from build123d import *

# Parameters (mm, degrees)
F0_W      = 6.5
F0_H      = 6.5
F1_DEPTH  = 34
F2_R      = 1
F4_DEPTH  = 8
F5_W      = 15
F5_H      = 15
F5_R      = 4
F6_DEPTH  = 10
F8_DEPTH  = 4
F10_D     = 4
F10_DEPTH = 25
F10_TIP   = 1.2017212381
F11_R     = 2


with BuildPart() as f1:
    # F0 (on Top) → F1 (new body)
    with BuildSketch(Plane.XY):
        Rectangle(F0_W, F0_H)
    extrude(amount=F1_DEPTH)

    # F2
    f2_edges = [f1.edges().sort_by_distance(p)[0] for p in [
        (-3.25, 3.25, 17),
        (3.25, 3.25, 17),
        (3.25, -3.25, 17),
        (-3.25, -3.25, 17),
    ]]
    fillet(f2_edges, radius=F2_R)

    # F3 (on face) → F4 (join)
    with BuildSketch(Plane.XY.offset(34)):
        with BuildLine():
            ThreePointArc((3.25, 2.25), (3.249048632, 2.2936099868), (3.2461963381, 2.3371369952))
            ThreePointArc((3.2461963381, 2.3371369952), (2.8284271247, 2.8284271247), (2.3371369952, 3.2461963381))
            ThreePointArc((2.3371369952, 3.2461963381), (2.2936099868, 3.249048632), (2.25, 3.25))
            Line((2.25, 3.25), (-2.25, 3.25))
            ThreePointArc((-2.25, 3.25), (-2.2936099868, 3.249048632), (-2.3371369952, 3.2461963381))
            ThreePointArc((-2.3371369952, 3.2461963381), (-2.8284271247, 2.8284271247), (-3.2461963381, 2.3371369952))
            ThreePointArc((-3.2461963381, 2.3371369952), (-3.249048632, 2.2936099868), (-3.25, 2.25))
            Line((-3.25, 2.25), (-3.25, -2.25))
            ThreePointArc((-3.25, -2.25), (-3.249048632, -2.2936099868), (-3.2461963381, -2.3371369952))
            ThreePointArc((-3.2461963381, -2.3371369952), (-2.8284271247, -2.8284271247), (-2.3371369952, -3.2461963381))
            ThreePointArc((-2.3371369952, -3.2461963381), (-2.2936099868, -3.249048632), (-2.25, -3.25))
            Line((-2.25, -3.25), (2.25, -3.25))
            ThreePointArc((2.25, -3.25), (2.2936099868, -3.249048632), (2.3371369952, -3.2461963381))
            ThreePointArc((2.3371369952, -3.2461963381), (2.8284271247, -2.8284271247), (3.2461963381, -2.3371369952))
            ThreePointArc((3.2461963381, -2.3371369952), (3.249048632, -2.2936099868), (3.25, -2.25))
            Line((3.25, -2.25), (3.25, 2.25))
        make_face()
        with BuildLine():
            ThreePointArc((3.2461963381, -2.3371369952), (3.8068875313, -1.2278466206), (4, 0))
            ThreePointArc((4, 0), (3.8068875313, 1.2278466206), (3.2461963381, 2.3371369952))
            ThreePointArc((3.2461963381, 2.3371369952), (3.249048632, 2.2936099868), (3.25, 2.25))
            Line((3.25, 2.25), (3.25, -2.25))
            ThreePointArc((3.25, -2.25), (3.249048632, -2.2936099868), (3.2461963381, -2.3371369952))
        make_face()
        with BuildLine():
            ThreePointArc((2.25, 3.25), (2.2936099868, 3.249048632), (2.3371369952, 3.2461963381))
            ThreePointArc((2.3371369952, 3.2461963381), (0, 4), (-2.3371369952, 3.2461963381))
            ThreePointArc((-2.3371369952, 3.2461963381), (-2.2936099868, 3.249048632), (-2.25, 3.25))
            Line((-2.25, 3.25), (2.25, 3.25))
        make_face()
        with BuildLine():
            ThreePointArc((-2.3371369952, -3.2461963381), (0, -4), (2.3371369952, -3.2461963381))
            ThreePointArc((2.3371369952, -3.2461963381), (2.2936099868, -3.249048632), (2.25, -3.25))
            Line((2.25, -3.25), (-2.25, -3.25))
            ThreePointArc((-2.25, -3.25), (-2.2936099868, -3.249048632), (-2.3371369952, -3.2461963381))
        make_face()
        with BuildLine():
            ThreePointArc((-3.25, 2.25), (-3.249048632, 2.2936099868), (-3.2461963381, 2.3371369952))
            ThreePointArc((-3.2461963381, 2.3371369952), (-4, 0), (-3.2461963381, -2.3371369952))
            ThreePointArc((-3.2461963381, -2.3371369952), (-3.249048632, -2.2936099868), (-3.25, -2.25))
            Line((-3.25, -2.25), (-3.25, 2.25))
        make_face()
    extrude(amount=F4_DEPTH)

    # F5 (on face) → F6 (join)
    with BuildSketch(Plane.XY.offset(42)):
        Rectangle(F5_W, F5_H)
        Circle(F5_R, mode=Mode.SUBTRACT)
        Circle(F5_R)
    extrude(amount=F6_DEPTH)

    # F7 (on face) → F8 (cut)
    with BuildSketch(Plane.XY.offset(52)):
        Polygon((-3, 1.7320508076), (-3, -1.7320508076), (0, -3.4641016151), (3, -1.7320508076), (3, 1.7320508076), (0, 3.4641016151), align=None)
    extrude(amount=-F8_DEPTH, mode=Mode.SUBTRACT)

    # F10
    with Locations(Plane.XY.offset(48)):
        with Locations((0, 0)):
            Hole(F10_D / 2, depth=F10_DEPTH)
            with Locations((0, 0, -(F10_DEPTH + F10_TIP / 2))):  # 118° drill point
                Cone(0, F10_D / 2, F10_TIP, mode=Mode.SUBTRACT)

    # F11
    f11_edges = [f1.edges().sort_by_distance(p)[0] for p in [
        (7.5, 7.5, 47),
        (-7.5, 7.5, 47),
        (-7.5, -7.5, 47),
        (7.5, -7.5, 47),
    ]]
    fillet(f11_edges, radius=F11_R)


solid = f1.part
Source: CAD feature listing. Evaluate the final solid. Frame: model axes, mm. A direction names the side the tool comes from. Give positions to 0.01 mm unless a question says otherwise; leave off trailing zeros. Write each loop counter-clockwise with the first axis right and the second up, starting at its lowest first coordinate (ties: lowest second). Pieces come first, ordered by that corner, then holes. Notation, with made-up numbers: (-38.5, -2) -> (-1.5, -2) arc R27 ccw to (-1.5, 37) -> close; hole circle Ø1 at (-27, 74). An arc over 180 degrees is marked (long way). Return JSON: item names as keys, results as strings. Group by question number.
1. Pin query (flat end, axial travel): pin 1 Ø3.5 at (x, z) = (-0.5, 12) entering from -Y; pin 2 Ø3.5 at (x, z) = (-0.5, 19) entering from +Y; pin 3 Ø0.6 at (x, y) = (-4, -0.5) entering from -Z. Return the tip coordinate at first contact, or that it passes through.
2. Section D-D, the plane y = 6.5. Output: boundary loops of the cut face in (x, z).
3. Section A-A, the plane z = 24. Output: boundary loops of the cut face in (x, y).
4. Mould query, pull axis X, two halves, no side actions, for faces 1 (the face through (-2.965, 2.949, 17.238)), 2 (the face through (0, 7.5, 47)), 3 (the face through (-0.08, -0.34, 22.01)). Classes: +X half, -X half, draft (parallel to the pull), parting line (faces both ways), or undercut.
5. Section B-B, the plane z = 8. Output: boundary loops of the cut face in (x, y).
6. Section C-C, the plane z = 35. Output: boundary loops of the cut face in (x, y), then the cut area to 3 significant figures.
7. Access query for faces 4 (the face through (0, 0, 0)), 5 (the face through (0, -3.25, 17)), 6 (the face through (2.965, 2.949, 17.238)), 7 (the face through (-2.965, -2.949, 17.238)), 8 (the face through (1.5, 2.6, 50)). Directions: +Z, -Z, +X, -X, +Y, -Y. A direction counts if a zero-diameter tool reaches every point of the face in a straight line with its end or side. Return the directions, or none.
8. Material intervals for line 1 (Y direction, x = 0, z = 31.25); line 2 (X direction, y = -1.5, z = 13), sorted ascending. Write a range as from..to.
Determined:
{
 "1": {"pin 1": "stops at y = -3.25", "pin 2": "stops at y = 3.25", "pin 3": "stops at z = 34"},
 "2": {"outline": "(-7.23, 42) -> (7.23, 42) -> (7.23, 52) -> (-7.23, 52) -> close"},
 "3": {"outline": "(-3.25, -2.25) arc R1 ccw to (-2.25, -3.25) -> (2.25, -3.25) arc R1 ccw to (3.25, -2.25) -> (3.25, 2.25) arc R1 ccw to (2.25, 3.25) -> (-2.25, 3.25) arc R1 ccw to (-3.25, 2.25) -> close; hole circle Ø4 at (0, 0)"},
 "4": {"face 1": "-X half", "face 2": "draft", "face 3": "undercut"},
 "5": {"outline": "(-3.25, -2.25) arc R1 ccw to (-2.25, -3.25) -> (2.25, -3.25) arc R1 ccw to (3.25, -2.25) -> (3.25, 2.25) arc R1 ccw to (2.25, 3.25) -> (-2.25, 3.25) arc R1 ccw to (-3.25, 2.25) -> close"},
 "6": {"outline": "circle Ø8 at (0, 0); hole circle Ø4 at (0, 0)", "area": "37.7 mm2"},
 "7": {"face 4": "-Z, +X, -X, +Y, -Y", "face 5": "-Z, +X, -X, -Y", "face 6": "-Z, +X, +Y", "face 7": "-Z, -X, -Y", "face 8": "+Z"},
 "8": {"line 1": "y = -3.25..-2, 2..3.25", "line 2": "x = -3.25..3.25"}
}
